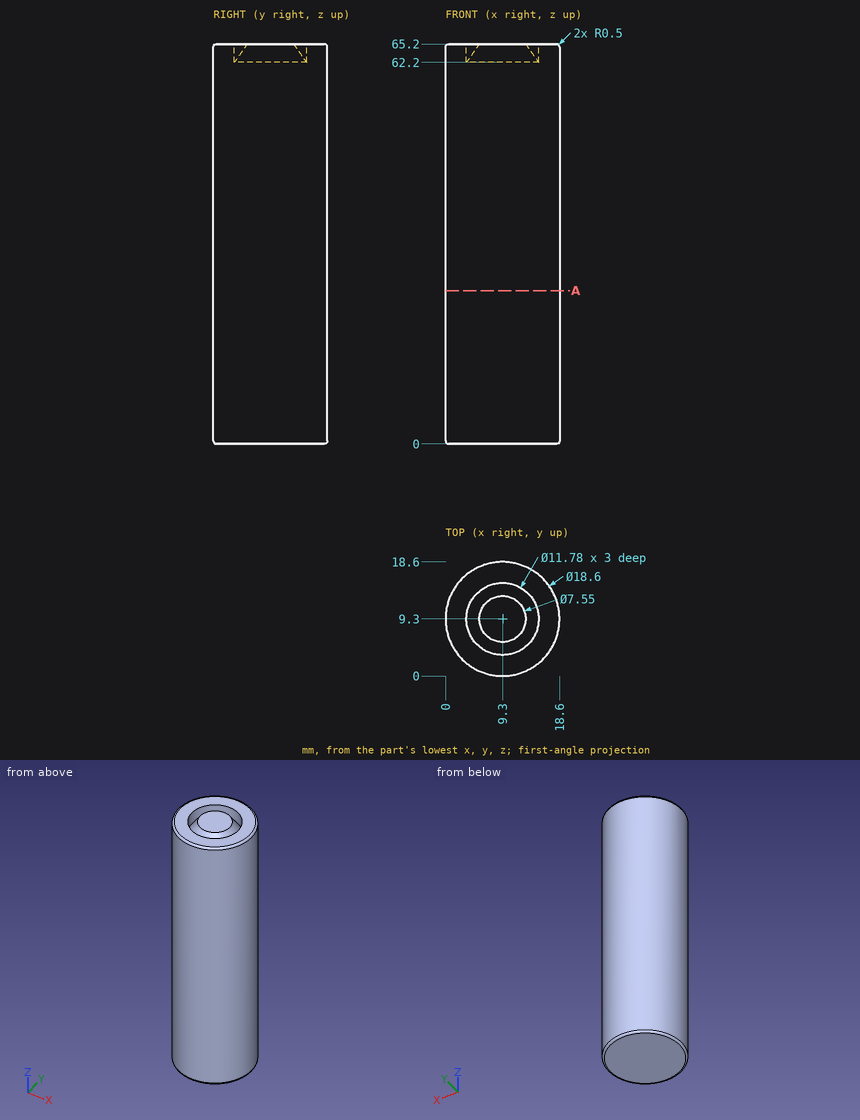
Study the drawing (mm; zero at the part's minimum x, y, z) and answer. Coordinates: 2 decimals unless noted, no trailing zeros. Write each loop counter-clockwise with the first axis right and the second up, starting at its lowest first coordinate (ties: lowest second). Pieces come first, ordered by that corner, then holes.
Q1. Find the intervals of material crossed by line 1 (X direction, y = 9.5, z = 13); line 2 (Y direction, x = 15, z = 30.5); line 3 (Y direction, x = 14.75, z = 51), in increasing order.
Q2. Each of these flat-tipped pins is pushed along its axis until it touches: pin 1 Ø2 at (y, z) = (5, 9) entering from -X; pin 2 Ø4 at (y, z) = (12.5, 47.5) entering from +X; pin 3 Ø2 at (x, z) = (4, 58) entering from +Y. Where does it stop, or does it pass through?
Q3. A cutting plane is placed at A-A, the plane z = 25. Give the vertices of the cut face in (x, y), then the cut area to 3 significant figures.
Findings below:
1. line 1: x = 0 to 18.6
1. line 2: y = 1.95 to 16.65
1. line 3: y = 1.76 to 16.84
2. pin 1: stops at x = 0.61
2. pin 2: stops at x = 18.52
2. pin 3: stops at y = 17.55
3. outline: circle Ø18.6 at (9.3, 9.3)
3. area: 272 mm2
